from build123d import *

# Parameters (mm, degrees)
F0_W     = 75.777124
F0_H     = 75.777124
F0_R     = 26.19375
F1_DEPTH = 14.2875
F2_R     = 30.95625
F3_DEPTH = 9.525
F4_R     = 0.79375


with BuildPart() as f1:
    # F0 (on Top) → F1 (new body)
    with BuildSketch(Plane.XY):
        Rectangle(F0_W, F0_H)
        Circle(F0_R, mode=Mode.SUBTRACT)
    extrude(amount=F1_DEPTH)

    # F2 (on Top) → F3 (cut)
    with BuildSketch(Plane.XY):
        Circle(F2_R)
    extrude(amount=F3_DEPTH, mode=Mode.SUBTRACT)

    # F4
    f4_edges = [f1.edges().sort_by_distance(p)[0] for p in [
        (-30.95625, 0, 9.525),
        (-37.888562, -37.888562, 7.14375),
        (37.888562, -37.888562, 7.14375),
        (37.888562, 37.888562, 7.14375),
        (-37.888562, 37.888562, 7.14375),
        (0, -37.888562, 14.2875),
        (-37.888562, 0, 14.2875),
        (0, 37.888562, 14.2875),
        (37.888562, 0, 14.2875),
    ]]
    fillet(f4_edges, radius=F4_R)


solid = f1.part
CAD build for the part. Positions are in the model's coordinates, mm. A direction names the side the tool comes from. Coordinates: 2 decimals unless noted, no trailing zeros. Loops run counter-clockwise (first coordinate to the right, second up) from the corner with the lowest first, then second, coordinate; pieces in that order, holes last. Notation, with made-up numbers: (-6.5, 29) - (38.5, 29) arc R29 cw to (38.5, 56) - close; hole circle Ø6 at (-28, -12). An arc over 180 degrees is marked (long way). Write item = value, one per line. Start each with the question number.
Q1. Cut at C-C, the plane z = 1.75. List the corners of the cut face in (x, y).
Q2. Cut at D-D, the plane z = 12. List the corners of the cut face in (x, y).
Q3. Which spindle directions (+Z, -Z, +X, -X, +Y, -Y) get a long thin tool onto all of the face, cutting with end or side? Do faces 1 (the flat face through (-17.4, 25.8, 0)), 2 (the cylindrical face through (-6.71, -30.22, 4.3)). Say none if no direction does.
Q4. Cut at A-A, the plane y = 0. List the corners of the cut face in (x, z) (1 decimal), then the cut area to 3 significant figures.
Q5. Drill centre lines: L1, parallel to Y at x = 0, z = 13.2; L2, parallel to X at y = -0.5, z = 1.75. Where is each one in solid material? Low to high.
Q6. Pull direction Y, two halves, no side cores. Call faces 3 (the flat face through (-1, 37.889, 7)), 4 (the flat face through (37.889, -1, 7)), 5 (the flat face through (-9, 25, 9.525)), 6 (the flat face through (-1, -37.889, 7)): pulls with the +Y half, pulls with the -Y half, needs draft (parallel to the pull), parting line crosses it, or undercut.
Computed:
q1.outline = (-37.89, -37.09) arc R0.79 ccw to (-37.09, -37.89) - (37.09, -37.89) arc R0.79 ccw to (37.89, -37.09) - (37.89, 37.09) arc R0.79 ccw to (37.09, 37.89) - (-37.09, 37.89) arc R0.79 ccw to (-37.89, 37.09) - close; hole circle Ø61.91 at (0, 0)
q2.outline = (-37.89, -37.09) arc R0.79 ccw to (-37.09, -37.89) - (37.09, -37.89) arc R0.79 ccw to (37.89, -37.09) - (37.89, 37.09) arc R0.79 ccw to (37.09, 37.89) - (-37.09, 37.89) arc R0.79 ccw to (-37.89, 37.09) - close; hole circle Ø52.39 at (0, 0)
q3.face_1 = -Z, +X, -X, +Y, -Y
q3.face_2 = -Z
q4.outline = (-37.9, 0) - (-31, 0) - (-31, 8.7) arc R0.8 cw to (-30.2, 9.5) - (-26.2, 9.5) - (-26.2, 14.3) - (-37.1, 14.3) arc R0.8 ccw to (-37.9, 13.5) - close; (26.2, 9.5) - (30.2, 9.5) arc R0.8 cw to (31, 8.7) - (31, 0) - (37.9, 0) - (37.9, 13.5) arc R0.8 ccw to (37.1, 14.3) - (26.2, 14.3) - close
q4.area = 243 mm²
q5.L1 = -37.89 to -26.19, 26.19 to 37.89
q5.L2 = -37.89 to -30.95, 30.95 to 37.89
q6.face_3 = pulls with the +Y half
q6.face_4 = needs draft
q6.face_5 = undercut
q6.face_6 = pulls with the -Y half
